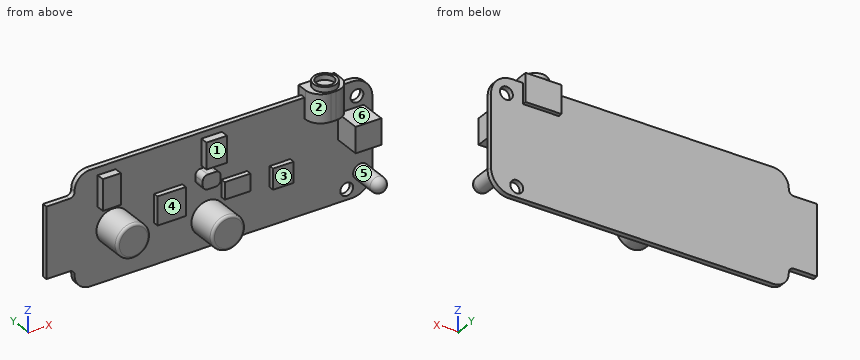
from build123d import *

# Parameters (mm, degrees)
SKETCH_1_R          = 1.25
EXTRUDE_1_DEPTH     = 1
SKETCH_2_R          = 1.5
EXTRUDE_2_DEPTH     = 6.5
FILLET_1_R          = 1.5
SKETCH_3_R          = 3.25
EXTRUDE_3_DEPTH     = 6
FILLET_2_R          = 0.5
SKETCH_4_W          = 5
SKETCH_4_H          = 5
EXTRUDE_4_DEPTH     = 5.2
SKETCH_5_W          = 4
SKETCH_5_H          = 4
SKETCH_5_W_2        = 5.5
SKETCH_5_H_2        = 5.5
SKETCH_5_W_3        = 5
SKETCH_5_H_3        = 3.3
EXTRUDE_5_DEPTH     = 1
SKETCH_6_W          = 3.5
SKETCH_6_H          = 2.8
EXTRUDE_6_DEPTH     = 2.2
FILLET_3_R          = 1
EXTRUDE_START       = -1.8
SKETCH_7_W          = 7
SKETCH_7_H          = 6.5
EXTRUDE_7_DEPTH     = 5
FILLET_4_R          = 3
SKETCH_8_R          = 2.25
SKETCH_8_R_2        = 1.75
CUT_EXTRUDE_1_DEPTH = 1
SKETCH_9_W          = 3.5
SKETCH_9_H          = 6
SKETCH_9_W_2        = 4
SKETCH_9_H_2        = 5.1
EXTRUDE_8_DEPTH     = 1.5


with BuildPart() as part:
    # Эскиз1 → Бобышка-Вытянуть1 (new body)
    with BuildSketch(Plane(origin=(0, 0, 0), x_dir=(1, 0, 0), z_dir=(0, 1, 0))):
        with BuildLine():
            Line((3, 0), (54, 0))
            ThreePointArc((54, 0), (56.828427125, 1.171572875), (58, 4))
            Line((58, 4), (58, 18))
            ThreePointArc((58, 18), (56.828427125, 20.828427125), (54, 22))
            Line((54, 22), (3, 22))
            ThreePointArc((3, 22), (0.878679656, 21.121320344), (0, 19))
            Line((0, 19), (0, 18.85))
            ThreePointArc((0, 18.85), (-0.292893219, 18.142893219), (-1, 17.85))
            Line((-1, 17.85), (-5.5, 17.85))
            Line((-5.5, 17.85), (-5.5, 4.15))
            Line((-5.5, 4.15), (-1, 4.15))
            ThreePointArc((-1, 4.15), (-0.292893219, 3.857106781), (0, 3.15))
            Line((0, 3.15), (0, 3))
            ThreePointArc((0, 3), (0.878679656, 0.878679656), (3, 0))
        make_face()
        with Locations(Location((53, 20, 0), (0, 0, 270))):
            Circle(SKETCH_1_R, mode=Mode.SUBTRACT)
        with Locations(Location((55, 3, 0), (0, 0, 270))):
            Circle(SKETCH_1_R, mode=Mode.SUBTRACT)
    extrude(amount=EXTRUDE_1_DEPTH)

    # Эскиз2 → Бобышка-Вытянуть2 (add)
    with BuildSketch(Plane.XZ):
        with Locations(Location((55.75, -17.5, 0), (0, 0, 90))):
            Circle(SKETCH_2_R)
    extrude(amount=EXTRUDE_2_DEPTH)

    # Скругление1
    fillet_1_edges = [part.edges().sort_by_distance(p)[0] for p in [
        (55.75, -6.5, -19),
    ]]
    fillet(fillet_1_edges, radius=FILLET_1_R)

    # Эскиз3 → Бобышка-Вытянуть3 (add)
    with BuildSketch(Plane.XZ):
        with Locations(Location((7.5, -12, 0), (0, 0, 90))):
            Circle(SKETCH_3_R)
        with Locations(Location((26, -16.5, 0), (0, 0, 90))):
            Circle(SKETCH_3_R)
    extrude(amount=EXTRUDE_3_DEPTH)

    # Скругление2
    fillet_2_edges = [part.edges().sort_by_distance(p)[0] for p in [
        (7.5, -6, -15.25),
        (26, -6, -19.75),
    ]]
    fillet(fillet_2_edges, radius=FILLET_2_R)

    # Эскиз4 → Бобышка-Вытянуть4 (add)
    with BuildSketch(Plane.XZ):
        with Locations((53.8, -7.6)):
            Rectangle(SKETCH_4_W, SKETCH_4_H)
    extrude(amount=EXTRUDE_4_DEPTH)

    # Эскиз5 → Бобышка-Вытянуть5 (add)
    with BuildSketch(Plane.XZ):
        with Locations((40, -12.7)):
            Rectangle(SKETCH_5_W, SKETCH_5_H)
        with Locations((18.25, -11.35)):
            Rectangle(SKETCH_5_W_2, SKETCH_5_H_2)
        with Locations((31.1, -11.85)):
            Rectangle(SKETCH_5_W_3, SKETCH_5_H_3)
    extrude(amount=EXTRUDE_5_DEPTH)

    # Эскиз6 → Бобышка-Вытянуть6 (add)
    with BuildSketch(Plane.XZ):
        with Locations((25.25, -8.2)):
            Rectangle(SKETCH_6_W, SKETCH_6_H)
    extrude(amount=EXTRUDE_6_DEPTH)

    # Скругление3
    fillet_3_edges = [part.edges().sort_by_distance(p)[0] for p in [
        (23.5, -1.1, -6.8),
        (23.5, -1.1, -9.6),
        (27, -1.1, -9.6),
        (27, -1.1, -6.8),
    ]]
    fillet(fillet_3_edges, radius=FILLET_3_R)

    # Эскиз7 → Бобышка-Вытянуть7 (add)
    with BuildSketch(Plane.XZ.offset(EXTRUDE_START)):
        with Locations((48.3, -0.75)):
            Rectangle(SKETCH_7_W, SKETCH_7_H)
    extrude(amount=EXTRUDE_7_DEPTH)

    # Скругление4
    fillet_4_edges = [part.edges().sort_by_distance(p)[0] for p in [
        (44.8, -3.2, -0.75),
        (51.8, -3.2, -0.75),
    ]]
    fillet(fillet_4_edges, radius=FILLET_4_R)

    # Эскиз8 → Вырез-Вытянуть1 (cut)
    # profile 1 of 2: a face of its own
    with BuildSketch(Plane.XY.offset(2.5)):
        with BuildLine():
            ThreePointArc((44.8, -0.2), (45.678679656, -2.321320344), (47.8, -3.2))
            Line((47.8, -3.2), (48.8, -3.2))
            ThreePointArc((48.8, -3.2), (50.921320344, -2.321320344), (51.8, -0.2))
            Line((51.8, -0.2), (51.8, 1.8))
            Line((51.8, 1.8), (44.8, 1.8))
            Line((44.8, 1.8), (44.8, -0.2))
        make_face()
        with Locations((48.3, -0.7)):
            Circle(SKETCH_8_R, mode=Mode.SUBTRACT)
    # profile 2 of 2: a face of its own
    with BuildSketch(Plane.XY.offset(2.5)):
        with Locations((48.3, -0.7)):
            Circle(SKETCH_8_R_2)
    extrude(amount=-CUT_EXTRUDE_1_DEPTH, mode=Mode.SUBTRACT)

    # Эскиз9 → Бобышка-Вытянуть8 (add)
    with BuildSketch(Plane.XZ):
        with Locations((6.25, -4.5)):
            Rectangle(SKETCH_9_W, SKETCH_9_H)
        with Locations((26.7, -3.75)):
            Rectangle(SKETCH_9_W_2, SKETCH_9_H_2)
    extrude(amount=EXTRUDE_8_DEPTH)


solid = part.part
Part model, mm, in its own coordinate system. Face numbers are marked on the shaded views. A direction names the side the tool comes from. Coordinates: 2 decimals unless noted, no trailing zeros. Order: outer loops, then holes, each group sorted by start corner. A loop starts at its lowest first (then second) coordinate and runs counter-clockwise, first axis right, second up.
(1) Slice it at C-C, the plane x = 18. Write the cut outline in (y, z), and give its area (3 significant figures).
Check sheet entries:
outline: (-1, -14.1) - (0, -14.1) - (0, -22) - (1, -22) - (1, 0) - (0, 0) - (0, -8.6) - (-1, -8.6) - close
area: 27.5 mm2
(2) Pin check, flat tips, straight feed: pin 1 Ø5 at (x, z) = (48, -14) entering from +Y; pin 2 Ø0.5 at (x, y) = (39, -0.5) entering from +Z; pin 3 Ø3 at (x, z) = (40, -13.5) entering from -Y; pin 4 Ø1.2 at (y, z) = (-0.5, -4) entering from -X. Stop position of each tip, or through.
Check sheet entries:
pin 1: stops at y = 1
pin 2: stops at z = -10.7
pin 3: stops at y = -1
pin 4: stops at x = -5.5
(3) Pull direction X, two halves, no side cores. Call the marked faces 4, 5 and 6: pulls with the +X half, pulls with the -X half, needs draft (parallel to the pull), parting line crosses it, or undercut.
Check sheet entries:
face 4: undercut
face 5: undercut
face 6: needs draft
(4) Slice it at A-A, the plane x = 53. Write the cut outline in (y, z).
Check sheet entries:
outline: (-5.2, -10.1) - (0, -10.1) - (0, -18.75) - (1, -18.75) - (1, 0) - (0, 0) - (0, -5.1) - (-5.2, -5.1) - close; (0, -22) - (1, -22) - (1, -21.25) - (0, -21.25) - close
(5) Tool access for the marked faces 1, 2 and 3: list every direction of +Z, -Z, +X, -X, +Y, -Y with a clear straight run to the whole face (end or side of a thin tool).
Check sheet entries:
face 1: +Z, -X, -Y
face 2: +Z, -Z, -Y
face 3: +Z, -Z, +X, -Y
(6) Slice it at B-B, the plane z = -12. Write the cut outline in (x, y).
Check sheet entries:
outline: (-5.5, 0) - (4.25, 0) - (4.25, -5.5) arc R0.5 ccw to (4.75, -6) - (10.25, -6) arc R0.5 ccw to (10.75, -5.5) - (10.75, 0) - (15.5, 0) - (15.5, -1) - (21, -1) - (21, 0) - (28.6, 0) - (28.6, -1) - (33.6, -1) - (33.6, 0) - (38, 0) - (38, -1) - (42, -1) - (42, 0) - (58, 0) - (58, 1) - (-5.5, 1) - close
(7) Probe L1, parallel to X at y = -0.75, z = -5.5; L2, parallel to Y at x = 10, z = -12.25; L3, parallel to Y at x = 35, z = -4. List the from-to ranges inside material, lowest first.
Check sheet entries:
L1: x = 4.5 to 8, 24.7 to 28.7, 51.3 to 56.3
L2: y = -6 to 1
L3: y = 0 to 1
